Design review of the part built by this model. Coordinates are the model's own, in mm. Face numbers are marked on the shaded views. A direction names the side the tool comes from. Coordinates: 2 decimals unless noted, no trailing zeros. Loops run counter-clockwise (first coordinate to the right, second up) from the corner with the lowest first, then second, coordinate; pieces in that order, holes last. Notation, with made-up numbers: (26, 19.5) -> (31, 19.5) arc R25 ccw to (31, 31.5) -> close; hole circle Ø4 at (-23, -12). An arc over 180 degrees is marked (long way). Use a Markdown table: item, result. Add a question column.
Q1. Take a section at A-A on y = 0. Write out the cut boundary in (x, z), plus the area to 3 significant figures.
Q2. For probe 1 along Z at (x, y) = (32.5, 0); probe 2 along X at (y, z) = (-2.75, 27); probe 3 along Y at (x, z) = (30.5, 3), list the stretches that pass through material, from the lowest coordinate up.
Q3. Take a section at C-C on z = -2.5. Write out the cut boundary in (x, y), plus the area to 3 significant figures.
Q4. Clearance check with flat-ended pins moving along their axes: pin 1 Ø16 at (y, z) = (0, 0) entering from -X; pin 2 Ø1 at (x, y) = (-12.5, 6) entering from +Z; pin 3 Ø10 at (x, z) = (40.5, -9) entering from +Y; pin 4 Ø5 at (x, y) = (41.5, 10) entering from +Z. State where each tip first meets the part, or that it passes through.
Q5. For the marked faces 1, 2 and 3, list the 3-axis set-ups (+Z, -Z, +X, -X, +Y, -Y) from which the entire face can be reached by the end or side of a thin tool; tool diameter is ignored.
Q6. Take a section at D-D on y = -5.5. Write out the cut boundary in (x, z), plus the area to 3 significant figures.
Q7. Take a section at B-B on x = 12.5. Write out the cut boundary in (y, z).
Q8. Draft analysis for pull direction Y (two halves, no side actions). For the marked faces 4, 5 and 6, state which applies: pulls with the +Y half, pulls with the -Y half, needs draft (parallel to the pull), parting line crosses it, or undercut.
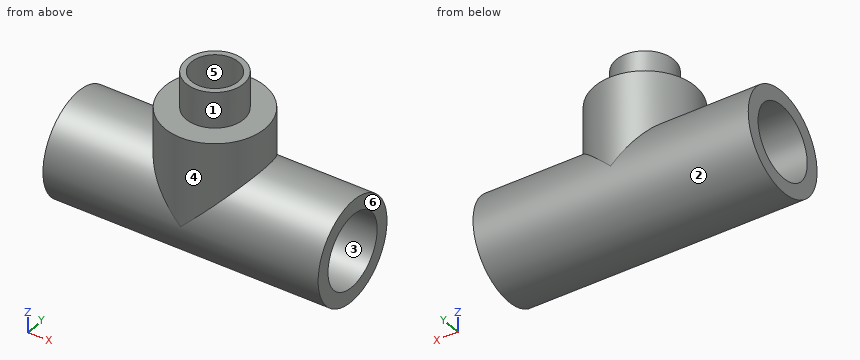
from build123d import *

# Parameters (mm, degrees)
F0_W     = 75
F0_H     = 4
F4_R     = 10
F5_DEPTH = 75.001


with BuildPart() as f1:
    # F0 (on Top) → F1 (revolve)
    with BuildSketch(Plane.XY):
        with Locations((12.5, 12)):
            Rectangle(F0_W, F0_H)
    revolve(axis=Axis((-0.954778, 0, 0), (1, 0, 0)))

    # F2 (on Front) → F3 (revolve)
    with BuildSketch(Plane.XZ):
        Polygon((-1.5, 25), (-1.5, 0), (6, 0), (6, 35), (4.5, 35), (4.5, 25), align=None)
    revolve(axis=Axis((12.5, 0, -7.054515), (0, 0, -1)))

    # F4 (on face) → F5 (cut, through all)
    with BuildSketch(Plane.YZ.offset(50)):
        Circle(F4_R)
    extrude(amount=-F5_DEPTH, mode=Mode.SUBTRACT)


solid = f1.part
Answer list:
| question | item | result |
|---|---|---|
| 1 | outline | (-25, -14) -> (50, -14) -> (50, -10) -> (-25, -10) -> close; (-25, 10) -> (50, 10) -> (50, 14) -> (26.5, 14) -> (26.5, 25) -> (20.5, 25) -> (20.5, 35) -> (19, 35) -> (19, 14) -> (6, 14) -> (6, 35) -> (4.5, 35) -> (4.5, 25) -> (-1.5, 25) -> (-1.5, 14) -> (-25, 14) -> close |
| 1 | area | 795 mm² |
| 2 | probe 1 | -14 to -10, 10 to 14 |
| 2 | probe 2 | 4.99 to 6.61, 18.39 to 20.01 |
| 2 | probe 3 | -13.67 to -9.54, 9.54 to 13.67 |
| 3 | outline | (-25, -13.77) -> (50, -13.77) -> (50, -9.68) -> (-25, -9.68) -> close; (-25, 9.68) -> (50, 9.68) -> (50, 13.77) -> (-25, 13.77) -> close |
| 3 | area | 614 mm² |
| 4 | pin 1 | through |
| 4 | pin 2 | z = 12.87 |
| 4 | pin 3 | y = 13.42 |
| 4 | pin 4 | z = 11.82 |
| 5 | face 1 | +Z |
| 5 | face 2 | none |
| 5 | face 3 | +X, -X |
| 6 | outline | (-25, -12.87) -> (50, -12.87) -> (50, -8.35) -> (-25, -8.35) -> close; (-25, 8.35) -> (50, 8.35) -> (50, 12.87) -> (25.37, 12.87) -> (25.37, 25) -> (18.31, 25) -> (18.31, 35) -> (15.96, 35) -> (15.96, 12.87) -> (9.04, 12.87) -> (9.04, 35) -> (6.69, 35) -> (6.69, 25) -> (-0.37, 25) -> (-0.37, 12.87) -> (-25, 12.87) -> close |
| 6 | area | 954 mm² |
| 7 | outline | (-14, 0) arc R14 ccw to (14, 0) -> (14, 25) -> (8, 25) -> (8, 35) -> (6.5, 35) -> (6.5, 12.4) arc R14 ccw to (-6.5, 12.4) -> (-6.5, 35) -> (-8, 35) -> (-8, 25) -> (-14, 25) -> close; hole circle Ø20 at (0, 0) |
| 8 | face 4 | parting line crosses it |
| 8 | face 5 | undercut |
| 8 | face 6 | needs draft |
